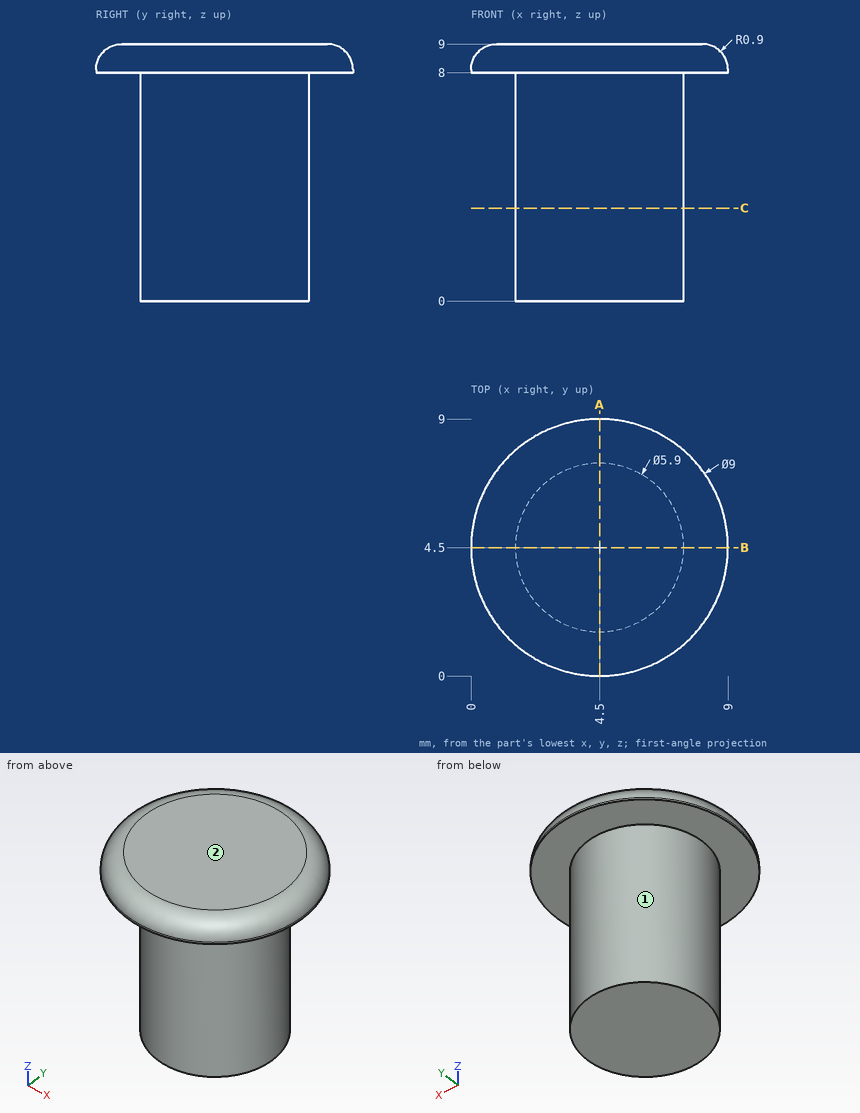
The figure shows three views and two pictorial views of one solid part (mm, origin at its lowest corner). Answer the questions. A direction names the side the tool comes from. Give positions to 0.01 mm unless a question says otherwise; leave off trailing zeros. Write each loop counter-clockwise with the first axis right and the second up, starting at its lowest first coordinate (ties: lowest second). Pieces come first, ordered by that corner, then holes. Notation, with made-up numbers: (-1, 78.25) - (9, 78.25) arc R27 cw to (9, 106.25) - close; hole circle Ø9 at (-0.75, 56). An arc over 180 degrees is marked (long way). Use CSV: the item, a comma, the result in double quotes. Start each with the question number.
Item 1: Consider line 1 (Z direction, x = 1.5, y = 4.25); line 2 (X direction, y = 4, z = 3.5); line 3 (X direction, y = 6, z = 5.5). Determine where each line is inside the solid, lowest interval first.
Item 2: The part is cut by section A-A, the plane x = 4.5. Give the vertices of the cut face in (y, z), and give its area (3 significant figures).
Item 3: The part is cut by section C-C, the plane z = 3.25. Give the vertices of the cut face in (x, y), and give its area (3 significant figures).
Item 4: Flat-ended cylindrical pins translate along their axes: P1, Ø3, axis at x = 5.5, z = 4, coming from the -Y side; P2, Ø1.5, axis at x = 7, z = 4.5, coming from the +Y side. Find the tip coordinate at first contact, or state that the pin passes through.
Item 5: For the marked faces 1 and 2, determine the directions among +Z, -Z, +X, -X, +Y, -Y from which every point of the face is accessible in a straight line to the end or side of a thin tool.
Taken from the geometry:
1,line 1,"8 to 9"
1,line 2,"1.59 to 7.41"
1,line 3,"1.96 to 7.04"
2,outline,"(0, 8) - (1.55, 8) - (1.55, 0) - (7.45, 0) - (7.45, 8) - (9, 8) - (9, 8.1) arc R0.9 ccw to (8.1, 9) - (0.9, 9) arc R0.9 ccw to (0, 8.1) - close"
2,area,"55.9 mm2"
3,outline,"circle Ø5.9 at (4.5, 4.5)"
3,area,"27.3 mm2"
4,P1,"y = 1.55"
4,P2,"y = 6.87"
5,face 1,"-Z"
5,face 2,"+Z, +X, -X, +Y, -Y"
